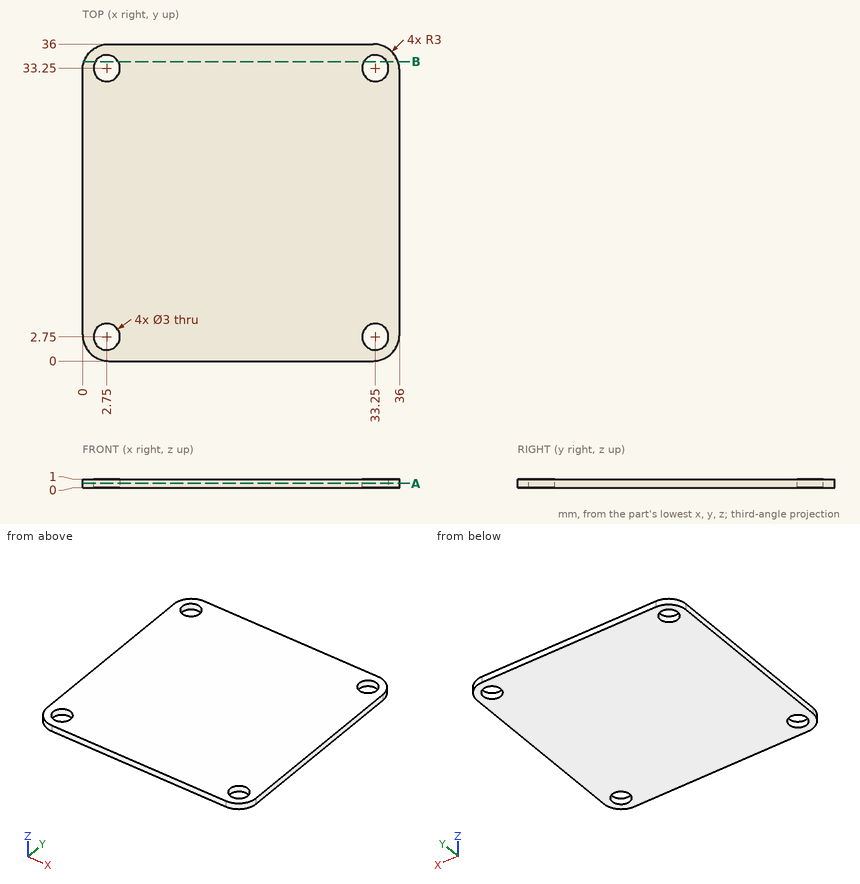
Part print with two shaded views. Sizes in mm from the minimum x, y, z corner. Coordinates: 2 decimals unless noted, no trailing zeros. Write each loop counter-clockwise with the first axis right and the second up, starting at its lowest first coordinate (ties: lowest second). Pieces come first, ordered by that corner, then holes. Notation, with made-up numbers: (-12.75, -39.5) -> (36.25, -39.5) arc R11 cw to (36.25, -33.5) -> close; hole circle Ø7 at (11, 50.5). An arc over 180 degrees is marked (long way). Return JSON: item names as keys, results as strings. Group by question number.
Q1. Cut at B-B, the plane y = 34. Give the cut face in (x, z), then the cut area to 3 significant figures.
Q2. Cut at A-A, the plane z = 0.5. Give the cut face in (x, y).
Q3. Drill centre lines: line 1 (Y direction, x = 33.25, z = 0.5); line 2 (Y direction, x = 34.5, z = 0.8); line 3 (X direction, y = 32.5, z = 0.45). Where is each one in solid material? Low to high.
Returned:
{
 "1": {"outline": "(0.17, 0) -> (1.45, 0) -> (1.45, 1) -> (0.17, 1) -> close; (4.05, 0) -> (31.95, 0) -> (31.95, 1) -> (4.05, 1) -> close; (34.55, 0) -> (35.83, 0) -> (35.83, 1) -> (34.55, 1) -> close", "area": "30.5 mm2"},
 "2": {"outline": "(0, 3) arc R3 ccw to (3, 0) -> (33, 0) arc R3 ccw to (36, 3) -> (36, 33) arc R3 ccw to (33, 36) -> (3, 36) arc R3 ccw to (0, 33) -> close; hole circle Ø3 at (2.75, 2.75); hole circle Ø3 at (2.75, 33.25); hole circle Ø3 at (33.25, 2.75); hole circle Ø3 at (33.25, 33.25)"},
 "3": {"line 1": "y = 0.01 to 1.25, 4.25 to 31.75, 34.75 to 35.99", "line 2": "y = 0.4 to 1.92, 3.58 to 32.42, 34.08 to 35.6", "line 3": "x = 0 to 1.45, 4.05 to 31.95, 34.55 to 36"}
}
